Here's how the part is built. I have some questions about the finished solid (model axes, mm). Face numbers are marked on the shaded views. A direction names the side the tool comes from. Coordinates: 2 decimals unless noted, no trailing zeros. Write each loop counter-clockwise with the first axis right and the second up, starting at its lowest first coordinate (ties: lowest second). Pieces come first, ordered by that corner, then holes.
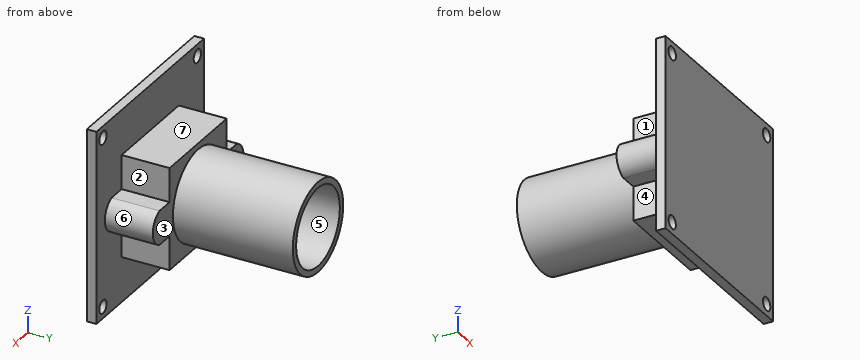
from build123d import *

# Parameters (mm, degrees)
SKETCH1_W            = 32
SKETCH1_H            = 32
PCB_THICKNESS_DEPTH  = 1.6
SKETCH2_W            = 17
SKETCH2_H            = 17
LENS_1_DEPTH         = 8
SKETCH3_R            = 7.5
LENS_2_DEPTH         = 20
LENS_3_DEPTH         = 8
SKETCH7_R            = 6.5
LENS_4_DEPTH         = 28
SKETCH5_R            = 1.1
MOUNTING_HOLES_DEPTH = 54.216538783


with BuildPart() as part:
    # Sketch1 → pcb_thickness (new body)
    with BuildSketch(Plane(origin=(0, 0, 0), x_dir=(1, 0, 0), z_dir=(0, 1, 0))):
        with Locations((-16, 16)):
            Rectangle(SKETCH1_W, SKETCH1_H)
    extrude(amount=PCB_THICKNESS_DEPTH)

    # Sketch2 → lens_1 (add)
    with BuildSketch(Plane(origin=(0, 1.6, 0), x_dir=(1, 0, 0), z_dir=(0, 1, 0))):
        with Locations((-16, 16)):
            Rectangle(SKETCH2_W, SKETCH2_H)
    extrude(amount=LENS_1_DEPTH)

    # Sketch3 → lens_2 (add)
    with BuildSketch(Plane(origin=(0, 9.6, 0), x_dir=(1, 0, 0), z_dir=(0, 1, 0))):
        with Locations(Location((-16, 16, 0), (0, 0, 270))):
            Circle(SKETCH3_R)
    extrude(amount=LENS_2_DEPTH)

    # Sketch6 → lens_3 (add)
    with BuildSketch(Plane(origin=(0, 1.6, 0), x_dir=(1, 0, 0), z_dir=(0, 1, 0))):
        with BuildLine():
            Line((-24.5, 18.828427125), (-27.5, 18.828427125))
            ThreePointArc((-27.5, 18.828427125), (-29.5, 16), (-27.5, 13.171572875))
            Line((-27.5, 13.171572875), (-24.5, 13.171572875))
            Line((-24.5, 13.171572875), (-24.5, 18.828427125))
        make_face()
        with BuildLine():
            Line((-7.5, 18.828427125), (-4.5, 18.828427125))
            ThreePointArc((-4.5, 18.828427125), (-2.5, 16), (-4.5, 13.171572875))
            Line((-4.5, 13.171572875), (-7.5, 13.171572875))
            Line((-7.5, 13.171572875), (-7.5, 18.828427125))
        make_face()
    extrude(amount=LENS_3_DEPTH)

    # Sketch7 → lens_4 (cut)
    with BuildSketch(Plane(origin=(0, 29.6, 0), x_dir=(1, 0, 0), z_dir=(0, 1, 0))):
        with Locations(Location((-16, 16, 0), (0, 0, 270))):
            Circle(SKETCH7_R)
    extrude(amount=-LENS_4_DEPTH, mode=Mode.SUBTRACT)

    # Sketch5 → mounting_holes (cut, through all)
    with BuildSketch(Plane(origin=(0, 1.6, 0), x_dir=(1, 0, 0), z_dir=(0, 1, 0))):
        with Locations(Location((-30.050000926, 30.050000926, 0), (0, 0, 270))):
            Circle(SKETCH5_R)
        with Locations(Location((-1.950000926, 30.049999074, 0), (0, 0, 270))):
            Circle(SKETCH5_R)
        with Locations(Location((-1.949999074, 1.949999074, 0), (0, 0, 270))):
            Circle(SKETCH5_R)
        with Locations(Location((-30.049999074, 1.950000926, 0), (0, 0, 270))):
            Circle(SKETCH5_R)
    extrude(amount=-MOUNTING_HOLES_DEPTH, mode=Mode.SUBTRACT)


solid = part.part
1. For pin 1 Ø3 at (x, z) = (-30.05, -1.95) entering from -Y; pin 2 Ø3 at (y, z) = (4, -20.5) entering from +X; pin 3 Ø6.5 at (x, y) = (-17, 7.5) entering from +Z; pin 4 Ø3 at (x, z) = (-15, -14) entering from +Y, each with a flat end and sliding along its axis, tell me the tip position at first contact or that it passes through.
2. I want a section at A-A (z = -1.95). List the corners of the cut face in (x, y) for me, then the cut area to 3 significant figures.
3. If I drill on line 1 (X direction, y = 1, z = -1.95); line 2 (X direction, y = 18, z = -16); line 3 (Y direction, x = -3.5, z = -22.5), over which ranges is the centre line in solid material (lowest first)?
4. I want a section at D-D (x = -10). List the corners of the cut face in (y, z) for me.
5. Thinking about a two-plate mould opening in Z: for the marked faces 5, 6 and 7, which applies, pulls with the +Z half, pulls with the -Z half, needs draft (parallel to the pull), parting line crosses it, or undercut?
6. I want a section at B-B (x = -30.05). List the corners of the cut face in (y, z) for me, then the cut area to 3 significant figures.
7. On a 3-axis mill with a long thin cutter (end or side, diameter ignored), from which of +Z, -Z, +X, -X, +Y, -Y can I reach the whole of each face in a straight line? I mean the marked faces 1, 2, 3 and 4. Say none if no direction works.
8. I want a section at C-C (y = 8.25). List the corners of the cut face in (x, z) for me, then the cut area to 3 significant figures.
Response values:
1. pin 1: stops at y = 0
1. pin 2: stops at x = -7.5
1. pin 3: stops at z = -7.5
1. pin 4: stops at y = 1.6
2. outline: (-32, 0) - (-31.15, 0) - (-31.15, 1.6) - (-32, 1.6) - close; (-28.95, 0) - (-3.05, 0) - (-3.05, 1.6) - (-28.95, 1.6) - close; (-0.85, 0) - (0, 0) - (0, 1.6) - (-0.85, 1.6) - close
2. area: 44.2 mm2
3. line 1: x = -32 to -31.15, -28.95 to -3.05, -0.85 to 0
3. line 2: x = -23.5 to -22.5, -9.5 to -8.5
3. line 3: y = 0 to 1.6
4. outline: (0, -32) - (1.6, -32) - (1.6, -24.5) - (9.6, -24.5) - (9.6, -20.5) - (29.6, -20.5) - (29.6, -18.5) - (1.6, -18.5) - (1.6, -13.5) - (29.6, -13.5) - (29.6, -11.5) - (9.6, -11.5) - (9.6, -7.5) - (1.6, -7.5) - (1.6, 0) - (0, 0) - close
5. face 5: undercut
5. face 6: parting line crosses it
5. face 7: pulls with the +Z half
6. outline: (0, -32) - (1.6, -32) - (1.6, -31.15) - (0, -31.15) - close; (0, -28.95) - (1.6, -28.95) - (1.6, -3.05) - (0, -3.05) - close; (0, -0.85) - (1.6, -0.85) - (1.6, 0) - (0, 0) - close
6. area: 44.2 mm2
7. face 1: +Z, -X, +Y
7. face 2: +Z, +X, +Y
7. face 3: +Y
7. face 4: -Z, -X, +Y
8. outline: (-27.5, -18.83) - (-24.5, -18.83) - (-24.5, -24.5) - (-7.5, -24.5) - (-7.5, -18.83) - (-4.5, -18.83) arc R3 ccw to (-4.5, -13.17) - (-7.5, -13.17) - (-7.5, -7.5) - (-24.5, -7.5) - (-24.5, -13.17) - (-27.5, -13.17) arc R3 ccw to start; hole circle Ø13 at (-16, -16)
8. area: 207 mm2
